```python
from build123d import *

# Parameters (mm, degrees)
CYLINDER001_R               = 3.5
CYLINDER001_DEPTH           = 280
CYLINDER001_ROLL_ANGLE      = 90
CYLINDER003_R               = 3.5
CYLINDER003_DEPTH           = 150
CYLINDER003_PITCH_ANGLE     = 90
CYLINDER003_PLACEMENT_ANGLE = 36
CYLINDER002_R               = 3.5
CYLINDER002_DEPTH           = 280
CYLINDER002_ROLL_ANGLE      = 90
CYLINDER004_R               = 3.5
CYLINDER004_DEPTH           = 150
CYLINDER004_PITCH_ANGLE     = 90
CYLINDER004_PLACEMENT_ANGLE = -36
CYLINDER005_R               = 3.5
CYLINDER005_DEPTH           = 150
CYLINDER006_R               = 3.5
CYLINDER006_DEPTH           = 384
CYLINDER006_PLACEMENT_ANGLE = 25
CYLINDER_R                  = 3.5
CYLINDER_DEPTH              = 560
CYLINDER_PITCH_ANGLE        = 90


with BuildPart() as obj1:
    # Cylinder001 → Cylinder001 (new body)
    with BuildSketch(Plane.XY):
        Circle(CYLINDER001_R)
    extrude(amount=CYLINDER001_DEPTH)


with BuildPart() as obj1_1:
    # Cylinder001 roll: moved
    add(obj1.part.rotate(Axis((0, 0, 0), (1, 0, 0)), CYLINDER001_ROLL_ANGLE))


with BuildPart() as obj1_2:
    # Cylinder001 placement: moved
    add(obj1_1.part.moved(Location((0, 140, 0))))


with BuildPart() as soporte_derecho:
    # Cylinder003 → Cylinder003 (new body)
    with BuildSketch(Plane.XY):
        Circle(CYLINDER003_R)
    extrude(amount=CYLINDER003_DEPTH)


with BuildPart() as soporte_derecho_1:
    # Cylinder003 pitch: moved
    add(soporte_derecho.part.rotate(Axis((0, 0, 0), (0, 1, 0)), CYLINDER003_PITCH_ANGLE))


with BuildPart() as soporte_derecho_2:
    # Cylinder003 placement: moved
    add(soporte_derecho_1.part.moved(Location((0, -90, 0))).rotate(Axis((0, -90, 0), (0, 0, 1)), CYLINDER003_PLACEMENT_ANGLE))


with BuildPart() as obj2:
    # Cylinder002 → Cylinder002 (new body)
    with BuildSketch(Plane.XY):
        Circle(CYLINDER002_R)
    extrude(amount=CYLINDER002_DEPTH)


with BuildPart() as obj2_1:
    # Cylinder002 roll: moved
    add(obj2.part.rotate(Axis((0, 0, 0), (1, 0, 0)), CYLINDER002_ROLL_ANGLE))


with BuildPart() as obj2_2:
    # Cylinder002 placement: moved
    add(obj2_1.part.moved(Location((560, 140, 0))))


with BuildPart() as soporte_izquierdo:
    # Cylinder004 → Cylinder004 (new body)
    with BuildSketch(Plane.XY):
        Circle(CYLINDER004_R)
    extrude(amount=CYLINDER004_DEPTH)


with BuildPart() as soporte_izquierdo_1:
    # Cylinder004 pitch: moved
    add(soporte_izquierdo.part.rotate(Axis((0, 0, 0), (0, 1, 0)), CYLINDER004_PITCH_ANGLE))


with BuildPart() as soporte_izquierdo_2:
    # Cylinder004 placement: moved
    add(soporte_izquierdo_1.part.moved(Location((0, 90, 0))).rotate(Axis((0, 90, 0), (0, 0, 1)), CYLINDER004_PLACEMENT_ANGLE))


with BuildPart() as obj3:
    # Cylinder005 → Cylinder005 (new body)
    with BuildSketch(Plane(origin=(188, 0, 0), x_dir=(1, 0, 0), z_dir=(0, 0, 1))):
        Circle(CYLINDER005_R)
    extrude(amount=CYLINDER005_DEPTH)


with BuildPart() as obj4:
    # Cylinder006 → Cylinder006 (new body)
    with BuildSketch(Plane.XY):
        Circle(CYLINDER006_R)
    extrude(amount=CYLINDER006_DEPTH)


with BuildPart() as obj4_1:
    # Cylinder006 placement: moved
    add(obj4.part.moved(Location((118, 0, 0))).rotate(Axis((118, 0, 0), (0, 1, 0)), CYLINDER006_PLACEMENT_ANGLE))


with BuildPart() as obj5:
    # Cylinder → Cylinder (new body)
    with BuildSketch(Plane.XY):
        Circle(CYLINDER_R)
    extrude(amount=CYLINDER_DEPTH)


with BuildPart() as obj5_1:
    # Cylinder pitch: moved
    add(obj5.part.rotate(Axis((0, 0, 0), (0, 1, 0)), CYLINDER_PITCH_ANGLE))


with BuildPart() as obj5_2:
    # Cylinder placement: moved
    add(obj5_1.part)

    # Fusion: union obj1, Soporte Derecho, obj2, Soporte Izquierdo, obj3, obj4
    add(obj1_2.part)
    add(soporte_derecho_2.part)
    add(obj2_2.part)
    add(soporte_izquierdo_2.part)
    add(obj3.part)
    add(obj4_1.part)


solid = obj5_2.part
```
Design review of the part built by this model. Coordinates are the model's own, in mm. Give positions to 0.01 mm unless a question says otherwise; leave off trailing zeros. Order: outer loops, then holes, each group sorted by start corner. A loop starts at its lowest first (then second) coordinate and runs counter-clockwise, first axis right, second up. Notation, with made-up numbers: (40, 54.5) -> (50, 54.5) arc R14 ccw to (50, 69.5) -> close; hole circle Ø1 at (58.25, 53). An arc over 180 degrees is marked (long way). Write item = value, one per line. Start each with the question number.
(1) Mouldability with a two-part tool opening along X and no side actions: class faces 1 (the face through (61.835, -49.298, 0.759)), 2 (the face through (201.376, 1.051, 170.901)) as +X half, -X half, draft (parallel to the pull), parting line (faces both ways), or undercut.
(2) To check wall thickness, follow line 1 along Z through (x, y) = (276, 1). State the ranges of the line that lie inside material, in increasing order.
(3) We need section B-B on y = -26. State how many separate pieces and enclosed holes the cut face has, plus the area to 3 significant figures.
(4) We need section A-A on x = 409. Write out the cut boundary in (y, z).
Numbers:
q1.face_1 = undercut
q1.face_2 = undercut
q2.line_1 = -3.35 to 3.35, 330.9 to 346.77
q3.separate_pieces = 3
q3.enclosed_holes = 0
q3.area = 142 mm^2
q4.outline = circle Ø7 at (0, 0)
